```python
from build123d import *

# Parameters (mm, degrees)
BOSS_EXTRUDE1_DEPTH = 22.225
SKETCH1_3_W         = 25.4
SKETCH1_3_H         = 38.1
BOSS_EXTRUDE2_DEPTH = 38.1
SKETCH1_4_W         = 25.4
SKETCH1_4_H         = 28.575
SKETCH1_4_H_2       = 34.925
BOSS_EXTRUDE3_DEPTH = 50.8
CUT_EXTRUDE1_DEPTH  = 25.4


with BuildPart() as part:
    # Sketch1 → Boss-Extrude1 (new body)
    with BuildSketch(Plane.XY):
        Polygon((25.4, 28.575), (25.4, 0), (88.9, 0), (88.9, 38.1), (57.15, 38.1), (57.15, 63.5), (25.4, 63.5), align=None)
    extrude(amount=BOSS_EXTRUDE1_DEPTH)

    # Sketch1_3 → Boss-Extrude2 (add)
    with BuildSketch(Plane.XY):
        with Locations((101.6, 19.05)):
            Rectangle(SKETCH1_3_W, SKETCH1_3_H)
    extrude(amount=BOSS_EXTRUDE2_DEPTH)

    # Sketch1_4 → Boss-Extrude3 (add)
    with BuildSketch(Plane.XY):
        with Locations((12.7, 14.2875)):
            Rectangle(SKETCH1_4_W, SKETCH1_4_H)
        with Locations((12.7, 46.0375)):
            Rectangle(SKETCH1_4_W, SKETCH1_4_H_2)
    extrude(amount=BOSS_EXTRUDE3_DEPTH)

    # Sketch2 → Cut-Extrude1 (cut)
    with BuildSketch(Plane.ZY):
        Polygon((50.8, 28.575), (30.636041849, 63.5), (50.8, 63.5), align=None)
    extrude(amount=-CUT_EXTRUDE1_DEPTH, mode=Mode.SUBTRACT)


solid = part.part
```
Can you work these out from the model? Positions are in its coordinate system, mm. A direction names the side the tool comes from. Coordinates: 2 decimals unless noted, no trailing zeros. Loops run counter-clockwise (first coordinate to the right, second up) from the corner with the lowest first, then second, coordinate; pieces in that order, holes last.
1) Imagine slicing it at A-A on z = 28. List the corners of the cut face in (x, y) for me, plus the area to 3 significant figures.
2) For pin 1 (18 mm diameter, centred on y = 54.5, z = 9, fed in from +X); pin 2 (2 mm diameter, centred on x = 63, y = 9, fed in from +Z) (3 decimals); pin 3 (20.5 mm diameter, centred on x = 98, y = 28.5, fed in from +Z), each with a flat end and sliding along its axis, tell me the tip position at first contact or that it passes through.
3) I need wall thicknesses on probe 1 along X at (y, z) = (32, 35); probe 2 along X at (y, z) = (12.5, 48.5); probe 3 along Y at (x, z) = (100, 13). Which ranges of each line are inside material? Lowest first, please.
4) Imagine slicing it at D-D on z = 18.5. List the corners of the cut face in (x, y) for me, plus the area to 3 significant figures.
5) Imagine slicing it at B-B on y = 24.5. List the corners of the cut face in (x, z) for me (3 decimals), plus the area to 3 significant figures.
6) Which directions (+Z, -Z, +X, -X, +Y, -Y) give clear straight access to the entire face, cutting with the end or side of a thin tool? Please do faces 4 (the flat face through (92, 38.1, 15)), 5 (the flat face through (101, 19, 38.1)), 6 (the flat face through (25.4, 24, 33)).
7) Imagine slicing it at C-C on x = 24. List the corners of the cut face in (y, z) for me (3 decimals).
8) Thinking about a two-plate mould opening in X: for faces 1 (the flat face through (114.3, 19, 19)), 2 (the flat face through (50, 25, 22.225)), 3 (the flat face through (28, 63.5, 15)), which applies, pulls with the +X half, pulls with the -X half, needs draft (parallel to the pull), parting line crosses it, or undercut?
Completed:
1. outline: (0, 0) - (25.4, 0) - (25.4, 63.5) - (0, 63.5) - close; (88.9, 0) - (114.3, 0) - (114.3, 38.1) - (88.9, 38.1) - close
1. area: 2,580 mm2
2. pin 1: stops at x = 57.15
2. pin 2: stops at z = 22.225
2. pin 3: stops at z = 38.1
3. probe 1: x = 0 to 25.4, 88.9 to 114.3
3. probe 2: x = 0 to 25.4
3. probe 3: y = 0 to 38.1
4. outline: (0, 0) - (114.3, 0) - (114.3, 38.1) - (57.15, 38.1) - (57.15, 63.5) - (0, 63.5) - close
4. area: 5,810 mm2
5. outline: (0, 0) - (114.3, 0) - (114.3, 38.1) - (88.9, 38.1) - (88.9, 22.225) - (25.4, 22.225) - (25.4, 50.8) - (0, 50.8) - close
5. area: 3,670 mm2
6. face 4: +Z, -Z, +X, +Y
6. face 5: +Z, +X, +Y, -Y
6. face 6: +Z, +Y, -Y
7. outline: (0, 0) - (63.5, 0) - (63.5, 30.636) - (28.575, 50.8) - (0, 50.8) - close
8. face 1: pulls with the +X half
8. face 2: undercut
8. face 3: needs draft
